The listing builds one solid part. Answer for the finished solid, in the listing's coordinates (mm). Round coordinates to 2 decimals unless told otherwise and drop trailing zeros. Write each loop counter-clockwise with the first axis right and the second up, starting at its lowest first coordinate (ties: lowest second). Pieces come first, ordered by that corner, then holes. Notation, with made-up numbers: (18, -25) - (51, -25) arc R31 cw to (51, 7) - close; hole circle Ø10 at (31, -17.5). An arc over 180 degrees is marked (long way). Answer in a Markdown table with one row per item.
from build123d import *

# Parameters (mm, degrees)
SKETCH1_W           = 103
SKETCH1_H           = 75
SKETCH1_W_2         = 24.25
SKETCH1_H_2         = 11.5
BOSS_EXTRUDE1_DEPTH = 4.5
SKETCH2_R           = 1.55
SCREWHOLES_DEPTH    = 64.865092187
SKETCH3_W           = 10.2
SKETCH3_H           = 4.7
BELTCLAMP_DEPTH     = 64.865092187
SKETCH4_W           = 10.2
SKETCH4_H           = 4.7
CUT_EXTRUDE3_DEPTH  = 64.865092187
SKETCH5_R           = 1.55
SKETCH5_W           = 4.7
SKETCH5_H           = 10.2
CUT_EXTRUDE4_DEPTH  = 64.865092187


with BuildPart() as part:
    # Sketch1 → Boss-Extrude1 (new body)
    with BuildSketch(Plane.XY):
        Rectangle(SKETCH1_W, SKETCH1_H)
        with Locations((-24.625, 22.5)):
            Rectangle(SKETCH1_W_2, SKETCH1_H_2, mode=Mode.SUBTRACT)
        with Locations((24.625, 22.5)):
            Rectangle(SKETCH1_W_2, SKETCH1_H_2, mode=Mode.SUBTRACT)
        with Locations((24.625, -22.5)):
            Rectangle(SKETCH1_W_2, SKETCH1_H_2, mode=Mode.SUBTRACT)
        with Locations((-24.625, -22.5)):
            Rectangle(SKETCH1_W_2, SKETCH1_H_2, mode=Mode.SUBTRACT)
    extrude(amount=BOSS_EXTRUDE1_DEPTH)

    # Sketch2 → screwHoles (cut, through all)
    with BuildSketch(Plane.XY.offset(4.5)):
        with Locations((-48, 33)):
            Circle(SKETCH2_R)
        with Locations(Location((48, 33, 0), (0, 0, 180))):
            Circle(SKETCH2_R)
        with Locations((40, 0)):
            Circle(SKETCH2_R)
        with Locations(Location((-40, 0, 0), (0, 0, 180))):
            Circle(SKETCH2_R)
        with Locations((0, 33)):
            Circle(SKETCH2_R)
    extrude(amount=-SCREWHOLES_DEPTH, mode=Mode.SUBTRACT)

    # Sketch3 → BeltClamp (cut, through all)
    with BuildSketch(Plane.XY.offset(4.5)):
        with Locations((-14, 9)):
            Rectangle(SKETCH3_W, SKETCH3_H)
        with Locations((14, 9)):
            Rectangle(SKETCH3_W, SKETCH3_H)
    extrude(amount=-BELTCLAMP_DEPTH, mode=Mode.SUBTRACT)

    # Sketch4 → Cut-Extrude3 (cut, through all)
    with BuildSketch(Plane.XY.offset(4.5)):
        Rectangle(SKETCH4_W, SKETCH4_H)
    extrude(amount=-CUT_EXTRUDE3_DEPTH, mode=Mode.SUBTRACT)

    # Sketch5 → Cut-Extrude4 (cut, through all)
    with BuildSketch(Plane.XY.offset(4.5)):
        with Locations((45, -31.75)):
            Circle(SKETCH5_R)
        with Locations(Location((-45, -31.75, 0), (0, 0, 180))):
            Circle(SKETCH5_R)
        with Locations((0, -31.75)):
            Circle(SKETCH5_R)
        with Locations((45, -9.75)):
            Rectangle(SKETCH5_W, SKETCH5_H)
        with Locations((-45, -9.75)):
            Rectangle(SKETCH5_W, SKETCH5_H)
    extrude(amount=-CUT_EXTRUDE4_DEPTH, mode=Mode.SUBTRACT)


solid = part.part
(1) Section A-A (x = 16.5) is taken. Give the vertices of the cut face in (y, z).
Checked values:
| item | result |
|---|---|
| outline | (-37.5, 0) - (-28.25, 0) - (-28.25, 4.5) - (-37.5, 4.5) - close; (-16.75, 0) - (6.65, 0) - (6.65, 4.5) - (-16.75, 4.5) - close; (11.35, 0) - (16.75, 0) - (16.75, 4.5) - (11.35, 4.5) - close; (28.25, 0) - (37.5, 0) - (37.5, 4.5) - (28.25, 4.5) - close |
(2) For a pull along Y with two mould halves and no side action, classify faces 1 (the flat face through (-1, -8, 0)), 2 (the cylindrical face through (-41.478, -0.466, 2.282)), 3 (the flat face through (-36.75, 22, 2)) as pulls with the +Y half, pulls with the -Y half, needs draft (parallel to the pull), parting line crosses it, or undercut.
Checked values:
| item | result |
|---|---|
| face 1 | needs draft |
| face 2 | undercut |
| face 3 | undercut |
(3) Section C-C (y = -25.5) is taken. Give the vertices of the cut face in (x, z).
Checked values:
| item | result |
|---|---|
| outline | (-51.5, 0) - (-36.75, 0) - (-36.75, 4.5) - (-51.5, 4.5) - close; (-12.5, 0) - (12.5, 0) - (12.5, 4.5) - (-12.5, 4.5) - close; (36.75, 0) - (51.5, 0) - (51.5, 4.5) - (36.75, 4.5) - close |
(4) Find the intervals of material crossed by line 1 (Y direction, x = 0, z = 2.6); line 2 (Y direction, x = -25.5, z = 4); line 3 (Y direction, x = -45, z = 2), in increasing order.
Checked values:
| item | result |
|---|---|
| line 1 | y = -37.5 to -33.3, -30.2 to -2.35, 2.35 to 31.45, 34.55 to 37.5 |
| line 2 | y = -37.5 to -28.25, -16.75 to 16.75, 28.25 to 37.5 |
| line 3 | y = -37.5 to -33.3, -30.2 to -14.85, -4.65 to 37.5 |
(5) Section B-B (y = 33) is taken. Give the vertices of the cut face in (x, z).
Checked values:
| item | result |
|---|---|
| outline | (-51.5, 0) - (-49.55, 0) - (-49.55, 4.5) - (-51.5, 4.5) - close; (-46.45, 0) - (-1.55, 0) - (-1.55, 4.5) - (-46.45, 4.5) - close; (1.55, 0) - (46.45, 0) - (46.45, 4.5) - (1.55, 4.5) - close; (49.55, 0) - (51.5, 0) - (51.5, 4.5) - (49.55, 4.5) - close |
(6) Section D-D (x = 45) is taken. Give the vertices of the cut face in (y, z), and give its area (3 significant figures).
Checked values:
| item | result |
|---|---|
| outline | (-37.5, 0) - (-33.3, 0) - (-33.3, 4.5) - (-37.5, 4.5) - close; (-30.2, 0) - (-14.85, 0) - (-14.85, 4.5) - (-30.2, 4.5) - close; (-4.65, 0) - (37.5, 0) - (37.5, 4.5) - (-4.65, 4.5) - close |
| area | 278 mm2 |
